```python
from build123d import *

# Parameters (mm, degrees)
CIRPATTERN1_COUNT    = 8
SKETCH10_W           = 4.2164
SKETCH10_H           = 38.1
BOSS_EXTRUDE1_DEPTH  = 25.4
FILLET1_R            = 5.08
SKETCH13_W           = 4.2164
SKETCH13_H           = 25.401
FILLET1_OF_MIRROR1_R = 5.08


with BuildPart() as part:
    # Sketch1 → Revolve2 (revolve)
    with BuildSketch(Plane.XY, mode=Mode.PRIVATE) as revolve2_sk:
        with BuildLine():
            Line((-63.5, 0), (-63.5, 63.5))
            Line((-63.5, 63.5), (-60.325, 63.5))
            Line((-60.325, 63.5), (-60.325, 38.1))
            Line((-60.325, 38.1), (-45.887987012, 38.1))
            ThreePointArc((-45.887987012, 38.1), (-37.592867218, 40.821117068), (-29.138150343, 42.996261447))
            ThreePointArc((-29.138150343, 42.996261447), (-17.316898362, 50.360212318), (-12.7, 63.5))
            Line((-12.7, 63.5), (-8.90651, 63.5))
            Line((-8.90651, 63.5), (-8.90651, 48.26))
            ThreePointArc((-8.90651, 48.26), (-11.993485386, 40.807382156), (-19.446103231, 37.720406769))
            ThreePointArc((-19.446103231, 37.720406769), (-32.858422717, 34.893706556), (-45.887987012, 30.638004221))
            ThreePointArc((-45.887987012, 30.638004221), (-54.721458819, 23.640172111), (-58.05478896, 12.875006597))
            Line((-58.05478896, 12.875006597), (-60.325, 0))
            Line((-60.325, 0), (-63.5, 0))
        make_face()
    revolve(revolve2_sk.sketch.rotate(Axis((0, 127.060987048, 0), (0, -1, 0)), 270), axis=Axis((0, 127.060987048, 0), (0, -1, 0)))

    # Sketch5 → #3 (0.213) Diameter Hole1 (revolve, cut)
    with BuildSketch(Plane(origin=(-24.300397955, 50.8, 58.666350314), x_dir=(0.9238795325112865, 0, 0.3826834323650904), z_dir=(0, 1, 0))):
        Polygon((0, 0), (0, 13.309388061), (2.7051, 11.684), (2.7051, 0), align=None)
    f_3_0_213_diameter_hole1 = revolve(axis=Axis((-26.730437751, 50.8, 64.532985346), (0.3826834323650904, 0, -0.9238795325112865)), mode=Mode.SUBTRACT)

    # CirPattern1: #3 (0.213) Diameter Hole1 ×8 about axis
    cirpattern1_axis = Axis((0, 127.060987048, 0), (0, -1, 0))
    for i in range(1, CIRPATTERN1_COUNT):
        add(f_3_0_213_diameter_hole1.rotate(cirpattern1_axis, i * 360 / CIRPATTERN1_COUNT), mode=Mode.SUBTRACT)

    # Sketch10 → Q (0.332) Diameter Hole2 (revolve, cut)
    with BuildSketch(Plane(origin=(-44.196, 38.1, 0), x_dir=(0, 0, 1), z_dir=(1, 0, 0))):
        with Locations((2.1082, 19.05)):
            Rectangle(SKETCH10_W, SKETCH10_H)
    revolve(axis=Axis((-44.196, 44.45, 0), (0, -1, 0)), mode=Mode.SUBTRACT)

    # Sketch11 → Boss-Extrude1 (add)
    with BuildSketch(Plane(origin=(0, 38.1, 0), x_dir=(1, 0, 0), z_dir=(0, 1, 0))):
        with BuildLine():
            Line((-59.841801652, 7.62), (-44.196, 7.62))
            ThreePointArc((-44.196, 7.62), (-36.576, -3.3653e-05), (-44.196067307, -7.62))
            Line((-44.196067307, -7.62), (-59.84181925, -7.619861803))
            ThreePointArc((-59.84181925, -7.619861803), (-60.325, 6.9657e-05), (-59.841801652, 7.62))
        make_face()
    boss_extrude1 = extrude(amount=BOSS_EXTRUDE1_DEPTH)

    # Fillet1
    fillet1_edges = [part.edges().sort_by_distance(p)[0] for p in [
        (-59.84181925, 50.8, 7.619861803),
        (-59.841801652, 50.8, -7.62),
    ]]
    fillet(fillet1_edges, radius=FILLET1_R)

    # Sketch13 → Q (0.332) Diameter Hole3 (revolve, cut)
    with BuildSketch(Plane(origin=(-44.196, 38.1, 0), x_dir=(0, 0, -1), z_dir=(1, 0, 0))):
        with Locations((2.1082, 12.7005)):
            Rectangle(SKETCH13_W, SKETCH13_H)
    q_0_332_diameter_hole3 = revolve(axis=Axis((-44.196, 31.75, 0), (0, 1, 0)), mode=Mode.SUBTRACT)

    # Mirror1: Boss-Extrude1, Q (0.332) Diameter Hole3 across plane
    add(boss_extrude1.mirror(Plane(origin=(0, 0, 0), x_dir=(0, 0, 1), z_dir=(1, 0, 0))))
    add(q_0_332_diameter_hole3.mirror(Plane(origin=(0, 0, 0), x_dir=(0, 0, 1), z_dir=(1, 0, 0))), mode=Mode.SUBTRACT)

    # Fillet1 of Mirror1
    fillet1_of_mirror1_edges = [part.edges().sort_by_distance(p)[0] for p in [
        (59.84181925, 50.8, 7.619861803),
        (59.841801652, 50.8, -7.62),
    ]]
    fillet(fillet1_of_mirror1_edges, radius=FILLET1_OF_MIRROR1_R)


solid = part.part
```
Could you check a few things on this model? Use its own coordinates, in mm. A direction names the side the tool comes from. Round coordinates to 2 decimals unless told otherwise and drop trailing zeros. Write each loop counter-clockwise with the first axis right and the second up, starting at its lowest first coordinate (ties: lowest second). Pieces come first, ordered by that corner, then holes. Notation, with made-up numbers: M 7.25,54 L 33.25,54 A23 ccw 33.25,78 Z; hole C 54.5,63 d8. An arc over 180 degrees is marked long. Answer in a Markdown table with one row per item. Add a question column.
Q1. Imagine slicing it at B-B (y = 26). Please give me the cut outline in (x, z), then the cut area to 3 significant figures.
Q2. If I drill on line 1 (X direction, y = 54.25, z = 0); line 2 (X direction, y = 55.5, z = 0); line 3 (X direction, y = 29, z = -4.5), over which ranges is the centre line in solid material (lowest first)? Write a range as from..to.
Q3. If we mould it in two halves opening along Y, with no side actions, what happens to faces 1 (the flat face through (37, 63.5, 0)), 2 (the cylindrical face through (-36.578, 50.812, -0.168)), 3 (the cylindrical face through (56.71, 53.2, -24.84)), 4 (the conical face through (51.6, 12.1, 26.9))? For each: +Y half, -Y half, draft (parallel to the pull), parting line (faces both ways), or undercut.
Q4. Will these pins go through, and if not, where does the flat tip stop? pin 1 Ø12 at (x, y) = (-8.5, 8) entering from +Z; pin 2 Ø5 at (x, z) = (-2.5, -23) entering from -Y; pin 3 Ø6 at (x, y) = (8.5, 43.5) entering from +Z; pin 4 Ø12 at (x, z) = (46, -50) entering from -Y.
Q5. Imagine slicing it at A-A (z = 0). Give the number of separate pieces and of enclosed holes in the cut face, then the cut area to 3 significant figures.
Q6. On a 3-axis mill with a long thin cutter (end or side, diameter ignored), from which of +Z, -Z, +X, -X, +Y, -Y can I reach the whole of each face in a straight line? I mean faces 5 (the cylindrical face through (57.71, 50.98, -9.5)), 6 (the cylindrical face through (56.97, 53.44, 24.23)). Say none if no direction works.
Values:
| question | item | result |
|---|---|---|
| 1 | outline | C 0,0 d127; hole C 0,0 d105.62 |
| 1 | area | 3,910 mm^2 |
| 2 | line 1 | -63.5..-48.41, -39.98..-36.58, -14.85..-8.91, 8.91..14.85, 36.58..39.98, 48.41..63.5 |
| 2 | line 2 | -63.5..-48.41, -39.98..-36.58, -14.28..-8.91, 8.91..14.28, 36.58..39.98, 48.41..63.5 |
| 2 | line 3 | -63.34..-48.94, 48.94..63.34 |
| 3 | face 1 | +Y half |
| 3 | face 2 | draft |
| 3 | face 3 | undercut |
| 3 | face 4 | -Y half |
| 4 | pin 1 | z = 63.45 |
| 4 | pin 2 | y = 36.6 |
| 4 | pin 3 | z = 63.26 |
| 4 | pin 4 | y = 0 |
| 5 | separate pieces | 3 |
| 5 | enclosed holes | 0 |
| 5 | area | 2,290 mm^2 |
| 6 | face 5 | +Y |
| 6 | face 6 | none |
